Part print with two shaded views. Sizes in mm from the minimum x, y, z corner. Round coordinates to 2 decimals unless told otherwise and drop trailing zeros. Loops run counter-clockwise (first coordinate to the right, second up) from the corner with the lowest first, then second, coordinate; pieces in that order, holes last. Notation, with made-up numbers: (-27.5, -24) - (21.5, -24) arc R34 cw to (21.5, 13) - close; hole circle Ø4 at (1, -32.5). An arc over 180 degrees is marked (long way). Use a Markdown table: item, result.
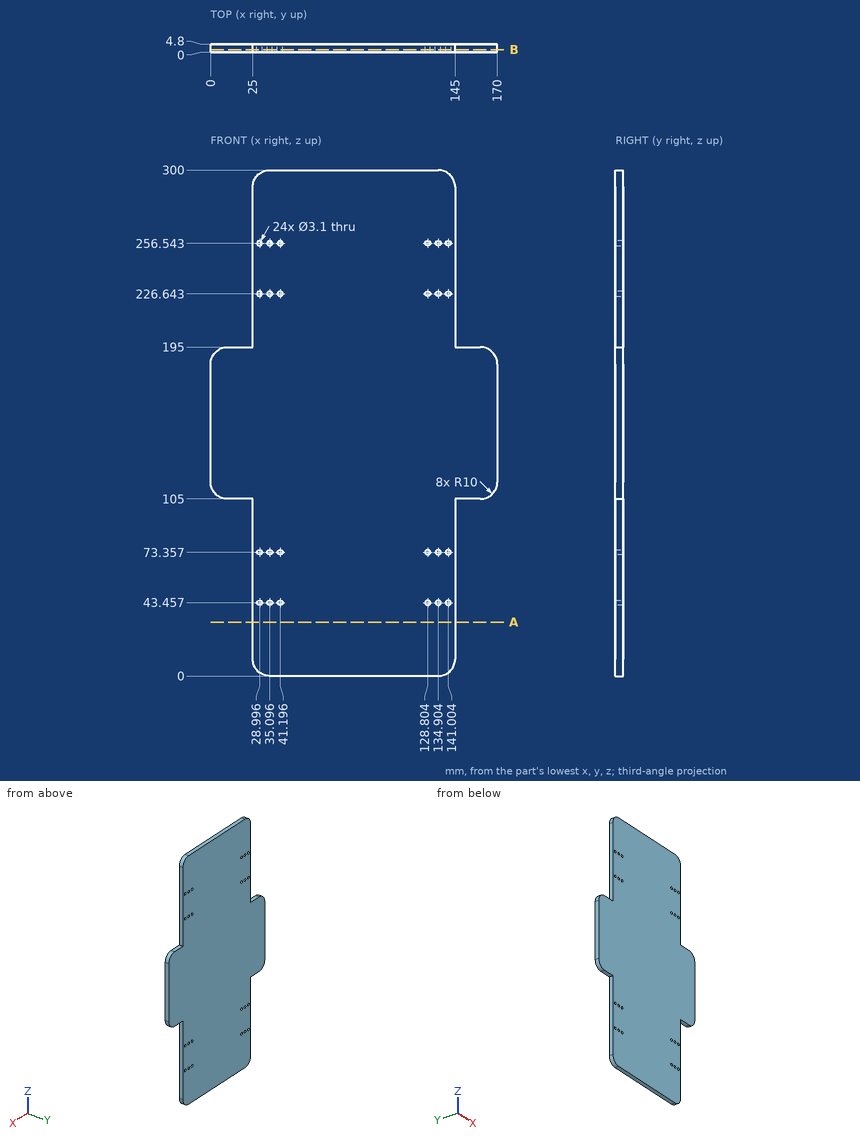
Q1. Probe line 1 (X direction, y = 2.1, z = 45.5); line 2 (Z direction, x = 155, y = 0.45). List the from-to ranges inside material, lowest first.
Results found:
| item | result |
|---|---|
| line 1 | x = 25 to 145 |
| line 2 | z = 105 to 195 |
Q2. Cut at B-B, the plane y = 1.45. Count the separate pieces of the cut face and the enclosed holes in it, plus the area to 3 significant figures.
Results found:
| item | result |
|---|---|
| separate pieces | 1 |
| enclosed holes | 24 |
| area | 40,100 mm2 |
Q3. Drop flat-ended pins along their axis: pin 1 (1.4 mm diameter, centred on x = 149, y = 2.5, fed in from +Z); pin 2 (1.4 mm diameter, centred on y = 1.5, z = 228.5, fed in from -X); pin 3 (2.5 mm diameter, centred on y = 2.5, z = 73.5, fed in from +X). Give the stop position or say it passes through.
Results found:
| item | result |
|---|---|
| pin 1 | stops at z = 195 |
| pin 2 | stops at x = 25 |
| pin 3 | stops at x = 145 |
Q4. Cut at A-A, the plane z = 32. List the corners of the cut face in (x, y), plus the area to 3 significant figures.
Results found:
| item | result |
|---|---|
| outline | (25, 0) - (145, 0) - (145, 4.8) - (25, 4.8) - close |
| area | 576 mm2 |
